```python
from build123d import *

# Parameters (mm, degrees)
SKETCH1_R           = 4.826
BOSS_EXTRUDE1_DEPTH = 95.25
CHAMFER1_SIZE       = 0.508
SKETCH4_W           = 0.9906
SKETCH4_H           = 0.9906


with BuildPart() as part:
    # Sketch1 → Boss-Extrude1 (new body)
    with BuildSketch(Plane.XY):
        Circle(SKETCH1_R)
    extrude(amount=BOSS_EXTRUDE1_DEPTH)

    # Chamfer1
    chamfer1_edges = [part.edges().sort_by_distance(p)[0] for p in [
        (-4.826, 0, 0),
        (-4.826, 0, 95.25),
    ]]
    chamfer(chamfer1_edges, length=CHAMFER1_SIZE)

    # Sketch4 → Cut-Revolve1 (revolve, cut)
    with BuildSketch(Plane(origin=(0, 0, 0), x_dir=(0, 0, -1), z_dir=(1, 0, 0)), mode=Mode.PRIVATE) as cut_revolve1_sk:
        with Locations((-3.7973, 4.3307)):
            Rectangle(SKETCH4_W, SKETCH4_H)
    revolve(cut_revolve1_sk.sketch.rotate(Axis((0, 0, -20.81511258), (0, 0, 1)), 90), axis=Axis((0, 0, -20.81511258), (0, 0, 1)), mode=Mode.SUBTRACT)


solid = part.part
```
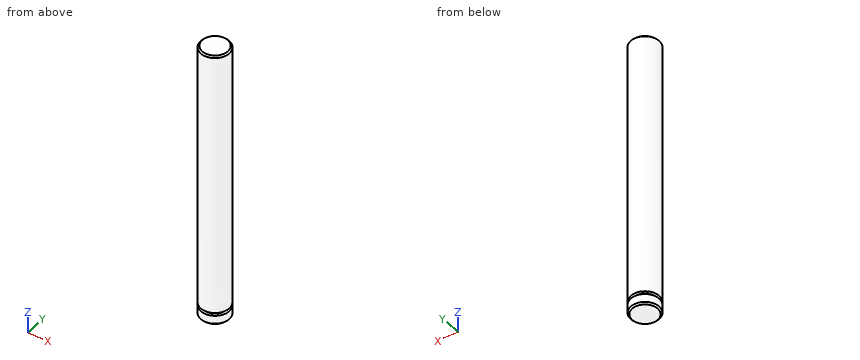
Design review of the part built by this model. Coordinates are the model's own, in mm. Coordinates: 2 decimals unless noted, no trailing zeros. Loops run counter-clockwise (first coordinate to the right, second up) from the corner with the lowest first, then second, coordinate; pieces in that order, holes last. Notation, with made-up numbers: (19.25, 43) -> (78.25, 43) arc R16 ccw to (78.25, 57) -> close; hole circle Ø2 at (32, 45). An arc over 180 degrees is marked (long way). Answer as a JSON object with one key per item and string values.
Q1. Take a section at A-A on z = 69. Give the boundary of the cut face in (x, y).
Answer block:
{"outline": "circle Ø9.65 at (0, 0)"}
Q2. Clearance check with flat-ended pins moving along their axes: pin 1 Ø4 at (y, z) = (2.5, 73.5) entering from +X; pin 2 Ø3 at (x, z) = (-3.5, 26.5) entering from +Y; pin 3 Ø3 at (x, y) = (-2, 2.5) entering from -Z; pin 4 Ø1.5 at (y, z) = (2, 81) entering from -X. State where each tip first meets the part, or that it passes through.
Answer block:
{"pin 1": "stops at x = 4.8", "pin 2": "stops at y = 4.39", "pin 3": "stops at z = 0", "pin 4": "stops at x = -4.66"}
Q3. To check wall thickness, follow L1, parallel to Z at x = -0.5, y = 4.25; L2, parallel to Z at x = -2.75, y = -3.5; L3, parallel to X at y = -0.25, z = 73. State the ranges of each line that lie inside material, in increasing order.
Answer block:
{"L1": "z = 0 to 3.3, 4.29 to 95.25", "L2": "z = 0.13 to 3.3, 4.29 to 95.12", "L3": "x = -4.82 to 4.82"}
